```python
from build123d import *

# Parameters (mm, degrees)
SKETCH1_R           = 1.524
BOSS_EXTRUDE1_DEPTH = 3.175
SKETCH2_R           = 1.524
CUT_EXTRUDE1_DEPTH  = 12.7
CHAMFER1_SIZE       = 1.905


with BuildPart() as part:
    # Sketch1 → Boss-Extrude1 (new body)
    with BuildSketch(Plane(origin=(0, 0, 0), x_dir=(1, 0, 0), z_dir=(0, 1, 0))):
        Polygon((-116.742050037, 65.586269915), (-116.742050037, -16.455730085), (-121.314050037, -16.455730085), (-121.314050037, -99.513730085), (-116.742050037, -99.513730085), (-116.742050037, -181.555730085), (-121.314050037, -181.555730085), (-213.770050037, -181.555730085), (-218.342050037, -181.555730085), (-218.342050037, -99.513730085), (-213.770050037, -99.513730085), (-213.770050037, -16.455730085), (-218.342050037, -16.455730085), (-218.342050037, 65.586269915), (-213.770050037, 65.586269915), (-213.770050037, 148.644269915), (-218.342050037, 148.644269915), (-218.342050037, 230.686269915), (-213.770050037, 230.686269915), (-213.770050037, 307.394269915), (-213.770050037, 313.744269915), (-121.314050037, 313.744269915), (-121.314050037, 307.394269915), (-121.314050037, 230.686269915), (-116.742050037, 230.686269915), (-116.742050037, 148.644269915), (-121.314050037, 148.644269915), (-121.314050037, 65.586269915), align=None)
        with Locations(Location((-119.028050037, 189.665269915, 0), (0, 0, 270))):
            Circle(SKETCH1_R, mode=Mode.SUBTRACT)
        with Locations(Location((-119.028050037, 24.565269915, 0), (0, 0, 270))):
            Circle(SKETCH1_R, mode=Mode.SUBTRACT)
        with Locations(Location((-119.028050037, -140.534730085, 0), (0, 0, 270))):
            Circle(SKETCH1_R, mode=Mode.SUBTRACT)
        with Locations(Location((-216.056050037, 189.665269915, 0), (0, 0, 90))):
            Circle(SKETCH1_R, mode=Mode.SUBTRACT)
        with Locations(Location((-216.056050037, 24.565269915, 0), (0, 0, 90))):
            Circle(SKETCH1_R, mode=Mode.SUBTRACT)
        with Locations(Location((-216.056050037, -140.534730085, 0), (0, 0, 90))):
            Circle(SKETCH1_R, mode=Mode.SUBTRACT)
        with Locations(Location((-167.542050037, -178.380730085, 0), (0, 0, 270))):
            Circle(SKETCH1_R, mode=Mode.SUBTRACT)
    extrude(amount=BOSS_EXTRUDE1_DEPTH)

    # Sketch2 → Cut-Extrude1 (cut)
    with BuildSketch(Plane.XZ):
        with Locations(Location((-168.088150037, -310.823269915, 0), (0, 0, 270))):
            Circle(SKETCH2_R)
    extrude(amount=-CUT_EXTRUDE1_DEPTH, mode=Mode.SUBTRACT)

    # Chamfer1
    # the kernel refuses this chamfer: 1.905 mm, written as the material it takes off along each edge
    with BuildSketch(Plane(origin=(-168.088150037, 0, -310.823269915), x_dir=(0, 0, -1), z_dir=(-1, 0, 0))) as chamfer1_piece_1:
        Polygon((1.524 + CHAMFER1_SIZE, 0), (1.524, -CHAMFER1_SIZE), (1.524, 0), align=None)
    revolve(axis=Axis((-168.088150037, 0, -310.823269915), (0, -1, 0)), mode=Mode.SUBTRACT)
    with BuildSketch(Plane(origin=(-119.028050037, 0, -189.665269915), x_dir=(0, 0, 1), z_dir=(-1, 0, 0))) as chamfer1_piece_2:
        Polygon((1.524 + CHAMFER1_SIZE, 0), (1.524, CHAMFER1_SIZE), (1.524, 0), align=None)
    revolve(axis=Axis((-119.028050037, 0, -189.665269915), (0, 1, 0)), mode=Mode.SUBTRACT)
    with BuildSketch(Plane(origin=(-119.028050037, 0, -24.565269915), x_dir=(0, 0, 1), z_dir=(-1, 0, 0))) as chamfer1_piece_3:
        Polygon((1.524 + CHAMFER1_SIZE, 0), (1.524, CHAMFER1_SIZE), (1.524, 0), align=None)
    revolve(axis=Axis((-119.028050037, 0, -24.565269915), (0, 1, 0)), mode=Mode.SUBTRACT)
    with BuildSketch(Plane(origin=(-216.056050037, 0, -189.665269915), x_dir=(0, 0, -1), z_dir=(1, 0, 0))) as chamfer1_piece_4:
        Polygon((1.524 + CHAMFER1_SIZE, 0), (1.524, CHAMFER1_SIZE), (1.524, 0), align=None)
    revolve(axis=Axis((-216.056050037, 0, -189.665269915), (0, 1, 0)), mode=Mode.SUBTRACT)
    with BuildSketch(Plane(origin=(-119.028050037, 0, 140.534730085), x_dir=(0, 0, 1), z_dir=(-1, 0, 0))) as chamfer1_piece_5:
        Polygon((1.524 + CHAMFER1_SIZE, 0), (1.524, CHAMFER1_SIZE), (1.524, 0), align=None)
    revolve(axis=Axis((-119.028050037, 0, 140.534730085), (0, 1, 0)), mode=Mode.SUBTRACT)
    with BuildSketch(Plane(origin=(-216.056050037, 0, -24.565269915), x_dir=(0, 0, -1), z_dir=(1, 0, 0))) as chamfer1_piece_6:
        Polygon((1.524 + CHAMFER1_SIZE, 0), (1.524, CHAMFER1_SIZE), (1.524, 0), align=None)
    revolve(axis=Axis((-216.056050037, 0, -24.565269915), (0, 1, 0)), mode=Mode.SUBTRACT)
    with BuildSketch(Plane(origin=(-216.056050037, 0, 140.534730085), x_dir=(0, 0, -1), z_dir=(1, 0, 0))) as chamfer1_piece_7:
        Polygon((1.524 + CHAMFER1_SIZE, 0), (1.524, CHAMFER1_SIZE), (1.524, 0), align=None)
    revolve(axis=Axis((-216.056050037, 0, 140.534730085), (0, 1, 0)), mode=Mode.SUBTRACT)
    with BuildSketch(Plane(origin=(-167.542050037, 0, 178.380730085), x_dir=(0, 0, 1), z_dir=(-1, 0, 0))) as chamfer1_piece_8:
        Polygon((1.524 + CHAMFER1_SIZE, 0), (1.524, CHAMFER1_SIZE), (1.524, 0), align=None)
    revolve(axis=Axis((-167.542050037, 0, 178.380730085), (0, 1, 0)), mode=Mode.SUBTRACT)


solid = part.part
```
Could you check a few things on this model? Use its own coordinates, in mm. Coordinates: 2 decimals unless noted, no trailing zeros. Write each loop counter-clockwise with the first axis right and the second up, starting at its lowest first coordinate (ties: lowest second). Pieces come first, ordered by that corner, then holes. Notation, with made-up numbers: (28, -22) -> (48, -22) arc R8 cw to (48, -14) -> close; hole circle Ø7 at (85.25, -6). An arc over 180 degrees is marked (long way). Write item = value, one per line. Start each with the question number.
(1) I want a section at A-A (y = 1.15). Give the number of separate pieces and of enclosed holes in the cut face, plus the area to 3 significant figures.
(2) Will this pin go through, and if not, where does the flat tip stop? pin 1 (1.6 mm diameter, centred on x = -119, y = 1, fed in from -Z).
(3) I want a section at B-B (z = 62). Please give me the cut outline in (x, y) (3 decimals), plus the area to 3 significant figures.
(4) I need wall thicknesses on line 1 (Z direction, x = -122, y = 0.1); line 2 (X direction, y = 1.9, z = -271.5). Which ranges of each line are inside material? Lowest first, please. Write a range as [from, to].
Result set:
q1.separate_pieces = 1
q1.enclosed_holes = 8
q1.area = 47,900 mm2
q2.pin_1 = -230.69
q3.outline = (-213.77, 0) -> (-121.314, 0) -> (-121.314, 3.175) -> (-213.77, 3.175) -> close
q3.area = 294 mm2
q4.line_1 = [-313.74, -191.17], [-188.17, -26.07], [-23.07, 139.03], [142.03, 181.56]
q4.line_2 = [-213.77, -121.31]
